from build123d import *

# Parameters (mm, degrees)
MODEL_R                 = 1.5
SALIENTE_EXTRUIR1_DEPTH = 3


with BuildPart() as part:
    # Model → Saliente-Extruir1 (new body)
    with BuildSketch(Plane.XY):
        with BuildLine():
            Line((21.294846678, 286.126884365), (18.742722334, 286.126884365))
            Line((18.742722334, 286.126884365), (18.742722334, 287.126884365))
            ThreePointArc((18.742722334, 287.126884365), (18.523052419, 287.657214451), (17.992722334, 287.876884365))
            Line((17.992722334, 287.876884365), (16.242722334, 287.876884365))
            ThreePointArc((16.242722334, 287.876884365), (15.712392248, 287.657214451), (15.492722334, 287.126884365))
            Line((15.492722334, 287.126884365), (15.492722334, 286.126884365))
            Line((15.492722334, 286.126884365), (9.201314468, 286.126884365))
            ThreePointArc((9.201314468, 286.126884365), (22.617722333, 298.126884365), (36.034130199, 286.126884365))
            Line((36.034130199, 286.126884365), (29.742722334, 286.126884365))
            Line((29.742722334, 286.126884365), (29.742722334, 287.126884365))
            ThreePointArc((29.742722334, 287.126884365), (29.523052419, 287.657214451), (28.992722334, 287.876884365))
            Line((28.992722334, 287.876884365), (27.242722334, 287.876884365))
            ThreePointArc((27.242722334, 287.876884365), (26.712392248, 287.657214451), (26.492722334, 287.126884365))
            Line((26.492722334, 287.126884365), (26.492722334, 286.126884365))
            Line((26.492722334, 286.126884365), (23.940597989, 286.126884365))
            ThreePointArc((23.940597989, 286.126884365), (22.617722333, 286.626884365), (21.294846678, 286.126884365))
        make_face()
        with Locations((22.617722334, 293.626884365)):
            Circle(MODEL_R, mode=Mode.SUBTRACT)
    extrude(amount=SALIENTE_EXTRUIR1_DEPTH)


solid = part.part
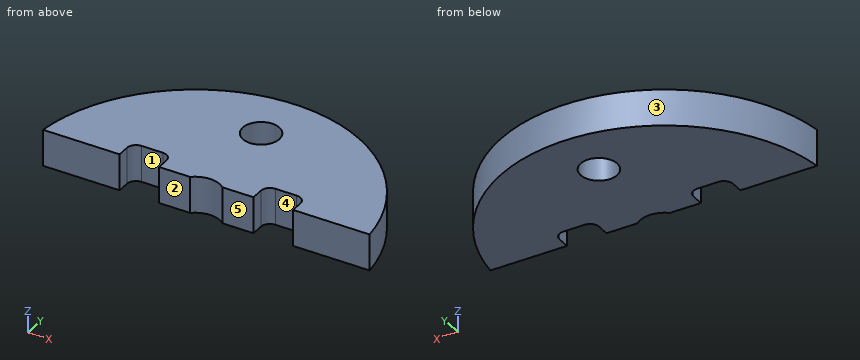
The model under review builds one solid part; all positions refer to its coordinate system, in mm. Face numbers are marked on the shaded views. A direction names the side the tool comes from. Round coordinates to 2 decimals unless told otherwise and drop trailing zeros. Order: outer loops, then holes, each group sorted by start corner. A loop starts at its lowest first (then second) coordinate and runs counter-clockwise, first axis right, second up. Notation, with made-up numbers: (32, -34) -> (53, -34) arc R31 cw to (53, 5) -> close; hole circle Ø1 at (-15, 55). An arc over 180 degrees is marked (long way). Return JSON: item names as keys, results as strings.
1. Take a section at C-C (y = 289.75). Write out the cut boundary in (x, z), then the cut area to 3 significant figures.
Answer block:
{"outline": "(10.13, 0) -> (35.11, 0) -> (35.11, 3) -> (10.13, 3) -> close", "area": "74.9 mm²"}
2. Take a section at B-B (z = 1.1). Write out the cut boundary in (x, y).
Answer block:
{"outline": "(9.2, 286.13) -> (15.49, 286.13) -> (15.49, 287.13) arc R0.75 cw to (16.24, 287.88) -> (17.99, 287.88) arc R0.75 cw to (18.74, 287.13) -> (18.74, 286.13) -> (21.29, 286.13) arc R2 cw to (23.94, 286.13) -> (26.49, 286.13) -> (26.49, 287.13) arc R0.75 cw to (27.24, 287.88) -> (28.99, 287.88) arc R0.75 cw to (29.74, 287.13) -> (29.74, 286.13) -> (36.03, 286.13) arc R13.5 ccw to start; hole circle Ø3 at (22.62, 293.63)"}
3. The part is to be moulded in two halves that separate along X. For the marked faces 1, 2 and 3, say which applies: +X half, -X half, draft (parallel to the pull), parting line (faces both ways), or undercut.
Answer block:
{"face 1": "undercut", "face 2": "draft", "face 3": "parting line"}
4. Insertion check: P1, Ø0.5, axis at y = 286.5, z = 2, coming from the -X side; P2, Ø0.5, axis at y = 287, z = 1.5, coming from the +X side; P3, Ø0.9, axis at x = 17.5, z = 1, coming from the -Y side. Each pin has a flat end and moves straight along its axis. Give the tip position at first contact, or say it passes through.
Answer block:
{"P1": "stops at x = 9.22", "P2": "stops at x = 35.95", "P3": "stops at y = 287.88"}
5. For L1, parallel to X at y = 287, z = 0.8; L2, parallel to X at y = 293, z = 1.45 (3 decimals); L3, parallel to X at y = 294, z = 2, list the stretches that pass through material, from the lowest coordinate up. Write a range as [from, to].
Answer block:
{"L1": "x = [9.33, 15.49], [18.74, 26.49], [29.74, 35.91]", "L2": "x = [12.028, 21.255], [23.98, 33.207]", "L3": "x = [12.9, 21.16], [24.07, 32.33]"}
6. For the marked faces 4 and 5, list the 3-axis set-ups (+Z, -Z, +X, -X, +Y, -Y) from which the entire face can be reached by the end or side of a thin tool; tool diameter is ignored.
Answer block:
{"face 4": "+Z, -Z, -Y", "face 5": "+Z, -Z, +X, -X, -Y"}
7. Take a section at A-A (x = 22.5). Write out the cut boundary in (y, z).
Answer block:
{"outline": "(286.62, 0) -> (292.13, 0) -> (292.13, 3) -> (286.62, 3) -> close; (295.12, 0) -> (298.13, 0) -> (298.13, 3) -> (295.12, 3) -> close"}
8. Take a section at D-D (x = 27.75). Write out the cut boundary in (y, z).
Answer block:
{"outline": "(287.88, 0) -> (297.11, 0) -> (297.11, 3) -> (287.88, 3) -> close"}
